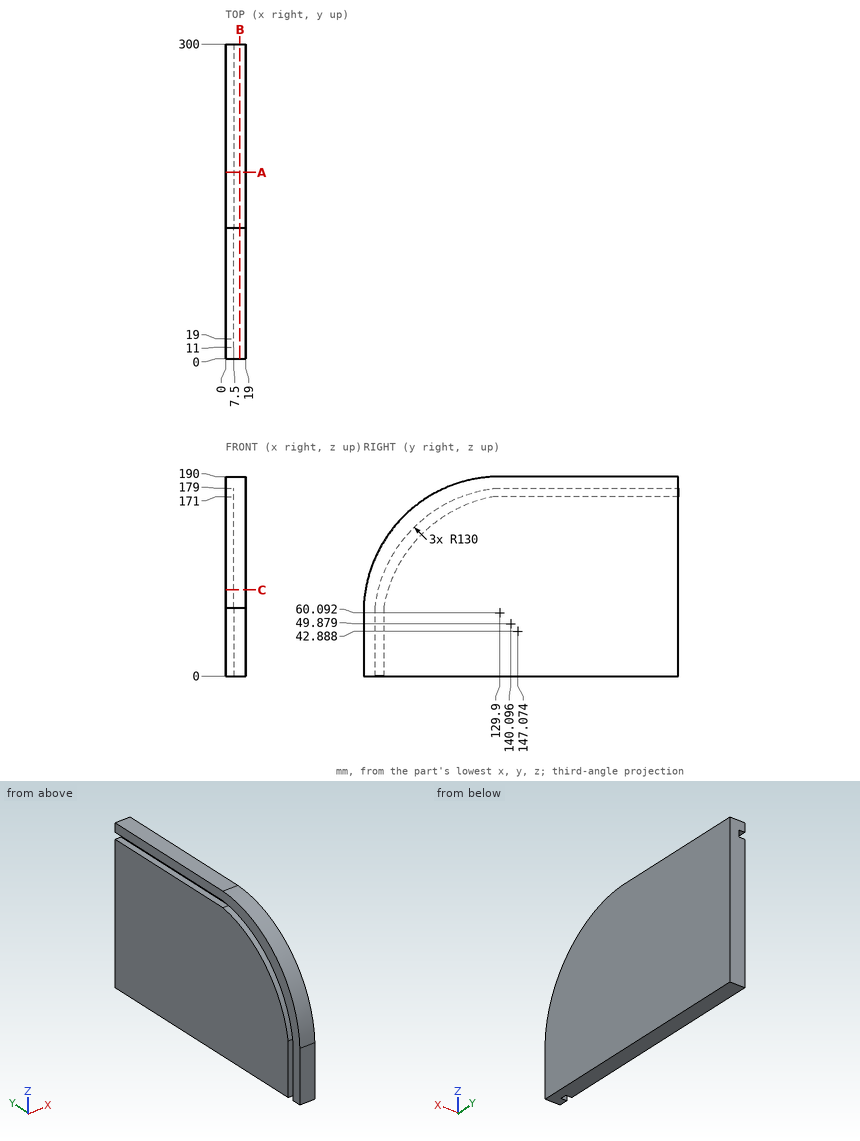
Design review of the part shown in the three views and the two pictorial views. Dimensions are in mm from the part's minimum x, y and z. Coordinates: 2 decimals unless noted, no trailing zeros. Order: outer loops, then holes, each group sorted by start corner. A loop starts at its lowest first (then second) coordinate and runs counter-clockwise, first axis right, second up.
1) Take a section at B-B, the plane x = 13.5. Give the boundary of the cut face in (y, z) (1 decimal), and give its area (3 significant figures).
2) Take a section at C-C, the plane z = 82. Give the boundary of the cut face in (x, y).
3) Clearance check with flat-ended pins moving along their axes: pin 1 (1.5 mm diameter, centred on x = 9, y = 104, fed in from +Z); pin 2 (6 mm diameter, centred on x = 9, y = 91, fed in from +Z); pin 3 (6 mm diameter, centred on x = 4, z = 148, fed in from -Y). State where each tip first meets the part, or that it passes through.
4) Take a section at A-A, the plane y = 177.5. Give the boundary of the cut face in (x, z).
5) Wall thickness on line 1 along Y through (x, z) = (5, 19.5); line 2 along Z through (x, y) = (6.75, 163.5); line 3 along Y through (x, z) = (4.25, 129) (1 decimal): over which ranges is each line inside the solid? List them lowest first.
Returned:
1. outline: (0, 0) - (300, 0) - (300, 190) - (125, 190) arc R130 ccw to (0, 65.2) - close
1. area: 53,400 mm2
2. outline: (0, 1.76) - (19, 1.76) - (19, 300) - (0, 300) - (0, 23.1) - (7.5, 23.1) - (7.5, 14.13) - (0, 14.13) - close
3. pin 1: stops at z = 187.64
3. pin 2: stops at z = 185.04
3. pin 3: stops at y = 31.46
4. outline: (0, 0) - (19, 0) - (19, 190) - (0, 190) - (0, 179) - (7.5, 179) - (7.5, 171) - (0, 171) - close
5. line 1: y = 0 to 11, 19 to 300
5. line 2: z = 0 to 171, 179 to 190
5. line 3: y = 19.7 to 36.9, 49.7 to 300
